Job drawing, mm, ordinate dimensions from the low corner. One solid piece. A direction names the side the tool comes from. Round coordinates to 2 decimals unless told otherwise and drop trailing zeros. Loops run counter-clockwise (first coordinate to the right, second up) from the corner with the lowest first, then second, coordinate; pieces in that order, holes last.
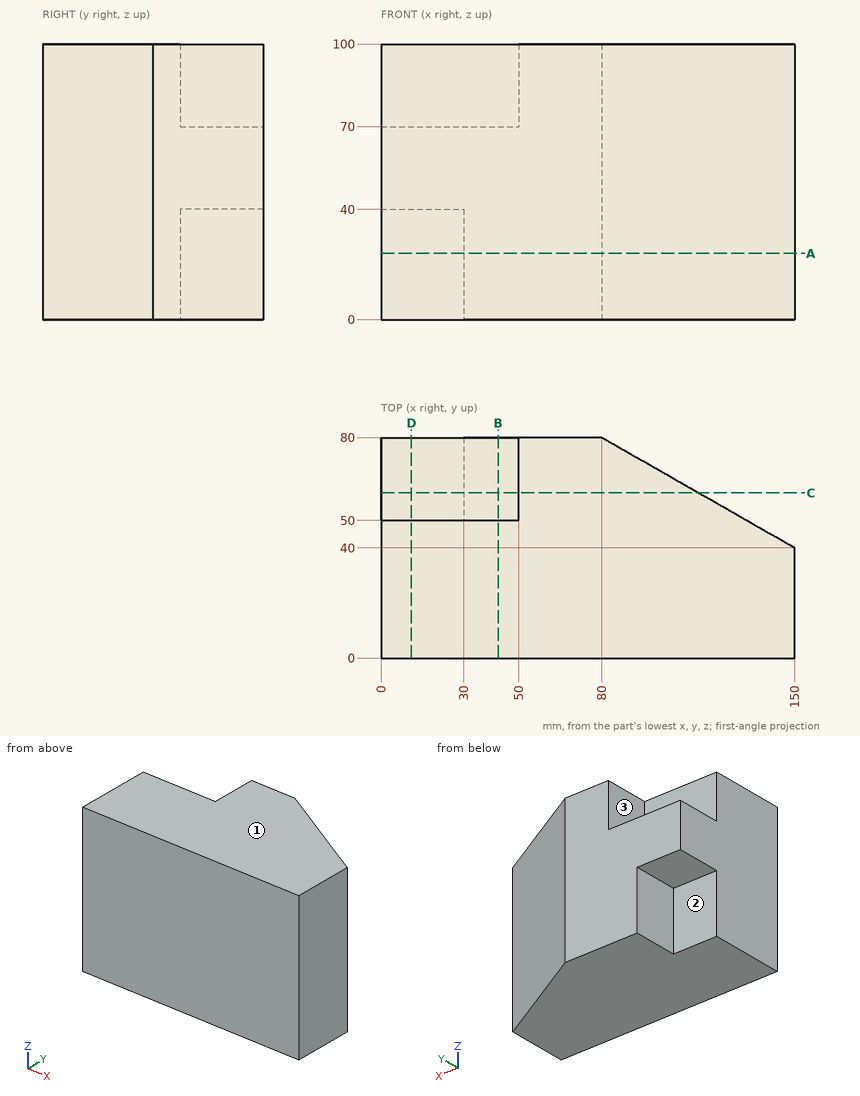
Item 1: Cut at D-D, the plane x = 11. Give the cut face in (y, z).
Answers follow:
outline: (0, 0) - (50, 0) - (50, 40) - (80, 40) - (80, 70) - (50, 70) - (50, 100) - (0, 100) - close
Item 2: Cut at C-C, the plane y = 60. Give the cut face in (x, z).
Answers follow:
outline: (0, 40) - (30, 40) - (30, 0) - (115, 0) - (115, 100) - (50, 100) - (50, 70) - (0, 70) - close
Item 3: Cut at A-A, the plane z = 24. Give the cut face in (x, y).
Answers follow:
outline: (0, 0) - (150, 0) - (150, 40) - (80, 80) - (30, 80) - (30, 50) - (0, 50) - close
Item 4: 3-axis set-ups, long thin cutter, end or side, ignore diameter. For the marked faces 1, 2 and 3: which of +Z, -Z, +X, -X, +Y, -Y reach the whole face in a straight line?
Answers follow:
face 1: +Z, +X, -X, +Y, -Y
face 2: -Z, -X, +Y
face 3: +Z, -X, +Y
Item 5: Cut at B-B, the plane x = 42.5. Give the cut face in (y, z), plus the area to 3 significant figures.
Answers follow:
outline: (0, 0) - (80, 0) - (80, 70) - (50, 70) - (50, 100) - (0, 100) - close
area: 7,100 mm2
Item 6: Flat gauge pins, fed straight in: P1, Ø2, axis at y = 65, z = 84.5, coming from the -X side; P2, Ø8, axis at x = 111, z = 30, coming from the +Y side; P3, Ø3, axis at y = 62.5, z = 53, coming from the +X side. Where does each tip first touch, or does it go through?
Answers follow:
P1: stops at x = 50
P2: stops at y = 64.57
P3: stops at x = 113.25
Item 7: Probe line 1 (Y direction, x = 18.5, z = 10); line 2 (Z direction, x = 8, y = 54); line 3 (Y direction, x = 99, z = 74.5). List the from-to ranges inside material, lowest first.
Answers follow:
line 1: y = 0 to 50
line 2: z = 40 to 70
line 3: y = 0 to 69.14
